Part model, mm, in its own coordinate system. A direction names the side the tool comes from. Coordinates: 2 decimals unless noted, no trailing zeros. Loops run counter-clockwise (first coordinate to the right, second up) from the corner with the lowest first, then second, coordinate; pieces in that order, holes last. Notation, with made-up numbers: (-26.5, 32.5) -> (-2.5, 32.5) arc R9 ccw to (-2.5, 43.5) -> close; hole circle Ø2 at (58.5, 33). An arc over 180 degrees is marked (long way). One line per item, written item: value. Start each with the question number.
from build123d import *

# Parameters (mm, degrees)
SKETCH6_R             = 3
BOSS_EXTRUDE4_DEPTH   = 4
BOSS_EXTRUDE4_2_DEPTH = 4
SKETCH7_R             = 2
CUT_EXTRUDE3_DEPTH    = 4
SKETCH8_W             = 3.845886706
SKETCH8_H             = 17
BOSS_EXTRUDE5_DEPTH   = 4
FILLET1_R             = 5
BOSS_EXTRUDE6_START   = -0.5
SKETCH9_R             = 2
BOSS_EXTRUDE6_DEPTH   = 0.5
SKETCH10_R            = 1.5
CUT_EXTRUDE4_DEPTH    = 0.5
BOSS_EXTRUDE7_START   = -0.5
SKETCH11_R            = 2
BOSS_EXTRUDE7_DEPTH   = 0.5
SKETCH12_R            = 1.5
CUT_EXTRUDE5_DEPTH    = 0.5


with BuildPart() as part:
    # Sketch6 → Boss-Extrude4 (new body)
    with BuildSketch(Plane.XY):
        Circle(SKETCH6_R)
    extrude(amount=BOSS_EXTRUDE4_DEPTH)


with BuildPart() as body_2:
    # Sketch6 → Boss-Extrude4 2 (new body)
    with BuildSketch(Plane.XY):
        with Locations((0, 21)):
            Circle(SKETCH6_R)
    extrude(amount=BOSS_EXTRUDE4_2_DEPTH)


with BuildPart() as cut_extrude3_tool:
    # Sketch7 → Cut-Extrude3 (new body)
    with BuildSketch(Plane.XY.offset(4)):
        with Locations((0, 21)):
            Circle(SKETCH7_R)
        Circle(SKETCH7_R)
    extrude(amount=-CUT_EXTRUDE3_DEPTH)


with BuildPart() as part_1:
    add(part.part)

    # Cut-Extrude3: cut by cut_extrude3_tool
    add(cut_extrude3_tool.part, mode=Mode.SUBTRACT)



with BuildPart() as body_2_1:
    add(body_2.part)

    # Cut-Extrude3: cut by cut_extrude3_tool
    add(cut_extrude3_tool.part, mode=Mode.SUBTRACT)


with BuildPart() as part_2:
    add(part_1.part)

    add(body_2_1.part)  # Boss-Extrude5 merges body 2
    # Sketch8 → Boss-Extrude5 (add)
    with BuildSketch(Plane.XY.offset(4)):
        with Locations((0, 10.5)):
            Rectangle(SKETCH8_W, SKETCH8_H)
    extrude(amount=-BOSS_EXTRUDE5_DEPTH)

    # Fillet1
    fillet1_edges = [part_2.edges().sort_by_distance(p)[0] for p in [
        (-1.922943353, 2.302669942, 2),
        (1.922943353, 2.302669942, 2),
        (1.922943353, 18.697330058, 2),
        (-1.922943353, 18.697330058, 2),
    ]]
    fillet(fillet1_edges, radius=FILLET1_R)

    # Sketch9 → Boss-Extrude6 (add)
    with BuildSketch(Plane(origin=(0, 0, 0), x_dir=(-1, 0, 0), z_dir=(0, 0, -1)).offset(BOSS_EXTRUDE6_START)):
        with Locations(Location((0, 21, 0), (0, 0, 180))):
            Circle(SKETCH9_R)
    extrude(amount=BOSS_EXTRUDE6_DEPTH)

    # Sketch10 → Cut-Extrude4 (cut)
    with BuildSketch(Plane.XY.offset(0.5)):
        with Locations((0, 21)):
            Circle(SKETCH10_R)
    extrude(amount=-CUT_EXTRUDE4_DEPTH, mode=Mode.SUBTRACT)

    # Sketch11 → Boss-Extrude7 (add)
    with BuildSketch(Plane(origin=(0, 0, 0), x_dir=(-1, 0, 0), z_dir=(0, 0, -1)).offset(BOSS_EXTRUDE7_START)):
        with Locations(Location((0, 0, 0), (0, 0, 180))):
            Circle(SKETCH11_R)
    extrude(amount=BOSS_EXTRUDE7_DEPTH)

    # Sketch12 → Cut-Extrude5 (cut)
    with BuildSketch(Plane.XY.offset(0.5)):
        Circle(SKETCH12_R)
    extrude(amount=-CUT_EXTRUDE5_DEPTH, mode=Mode.SUBTRACT)


solid = part_2.part
1) Probe line 1 (Y direction, x = 0, z = 0.25); line 2 (Y direction, x = 0, z = 2.4); line 3 (Y direction, x = -2.6, z = 3.7). List the from-to ranges inside material, lowest first. Write a range as from..to.
2) Slice it at D-D (y = 11.75). Give the cut face in (x, z), then the cut area to 3 significant figures.
3) Tool access for faces 3 (the cylindrical face through (-2.09, 2.73, 1.97)), 4 (the cylindrical face through (2.09, 2.73, 1.97)), 5 (the cylindrical face through (0, -2, 2)): list every direction of +Z, -Z, +X, -X, +Y, -Y with a clear straight run to the whole face (end or side of a thin tool).
4) Pull direction Y, two halves, no side cores. Call faces 1 (the flat face through (-1.923, 10, 2)), 2 (the flat face through (0, 11, 4)): +Y half, -Y half, draft (parallel to the pull), parting line (faces both ways), or undercut.
5) Pin check, flat tips, straight feed: pin 1 Ø1.8 at (x, y) = (0, 0) entering from -Z; pin 2 Ø1.2 at (y, z) = (9, 2.5) entering from +X; pin 3 Ø2 at (x, y) = (1, 6) entering from -Z; pin 4 Ø1.2 at (x, y) = (1, 20.5) entering from +Z. Stop position of each tip, or through.
6) Slice it at B-B (z = 2.4). Give the cut face in (x, y), then the cut area to 3 significant figures.
7) Slice it at C-C (x = -0.75). Give the cut face in (y, z), then the cut area to 3 significant figures.
8) Slice it at A-A (y = 0). Give the cut face in (x, z), then the cut area to 3 significant figures.
Check sheet entries:
1. line 1: y = -3..-1.5, 1.5..19.5, 22.5..24
1. line 2: y = -3..-2, 2..19, 23..24
1. line 3: y = -1.5..1.5, 19.5..22.5
2. outline: (-1.92, 0) -> (1.92, 0) -> (1.92, 4) -> (-1.92, 4) -> close
2. area: 15.4 mm^2
3. face 3: +Z, -Z, -X
3. face 4: +Z, -Z, +X
3. face 5: +Z
4. face 1: undercut
4. face 2: draft
5. pin 1: passes through
5. pin 2: stops at x = 1.92
5. pin 3: stops at z = 0
5. pin 4: stops at z = 0.5
6. outline: (-2.6, 1.5) arc R3 ccw (long way) to (2.6, 1.5) arc R5 cw to (1.92, 4.01) -> (1.92, 16.99) arc R5 cw to (2.6, 19.5) arc R3 ccw (long way) to (-2.6, 19.5) arc R5 cw to (-1.92, 16.99) -> (-1.92, 4.01) arc R5 cw to start; hole circle Ø4 at (0, 0); hole circle Ø4 at (0, 21)
6. area: 91.8 mm^2
7. outline: (-2.9, 0) -> (-1.3, 0) -> (-1.3, 0.5) -> (-1.85, 0.5) -> (-1.85, 4) -> (-2.9, 4) -> close; (1.3, 0) -> (19.7, 0) -> (19.7, 0.5) -> (19.15, 0.5) -> (19.15, 4) -> (1.85, 4) -> (1.85, 0.5) -> (1.3, 0.5) -> close; (22.3, 0) -> (23.9, 0) -> (23.9, 4) -> (22.85, 4) -> (22.85, 0.5) -> (22.3, 0.5) -> close
7. area: 78.7 mm^2
8. outline: (-3, 0) -> (-1.5, 0) -> (-1.5, 0.5) -> (-2, 0.5) -> (-2, 4) -> (-3, 4) -> close; (1.5, 0) -> (3, 0) -> (3, 4) -> (2, 4) -> (2, 0.5) -> (1.5, 0.5) -> close
8. area: 8.50 mm^2
